Work out the finished part from the listing and answer in its coordinate system (mm). Round coordinates to 2 decimals unless told otherwise and drop trailing zeros. Write each loop counter-clockwise with the first axis right and the second up, starting at its lowest first coordinate (ties: lowest second). Pieces come first, ordered by that corner, then holes.
1. Find section B-B (x = 14). Write down the section's boundary in (y, z), and give its area (3 significant figures).
2. Straight lines are drawn through the part: probe 1 along Y at (x, z) = (0, -0.9); probe 2 along Y at (x, z) = (9, 0.9); probe 3 along Y at (x, z) = (-5.5, -1.25). For each, find the intervals that lie inside material, in ascending order.
3. Find section A-A (z = -0.25). Write down the section's boundary in (x, y).
4. Flat-ended cylindrical pins translate along their axes: pin 1 Ø1.5 at (y, z) = (-187.5, -0.5) entering from +X; pin 2 Ø1 at (x, z) = (7.5, 0.5) entering from +Y; pin 3 Ø1.5 at (x, z) = (12, 0) entering from -Y. Find the tip coordinate at first contact, or state that the pin passes through.
Autodesk Inventor part; units mm, degrees
ref_plane "YZ Plane" through (0, 0, 0) normal (1, 0, 0) x (0, 1, 0)
ref_plane "XZ Plane" through (0, 0, 0) normal (0, 1, 0) x (-1, 0, 0)
ref_plane "XY Plane" through (0, 0, 0) normal (0, 0, 1) x (1, 0, 0)
sketch "Sketch1" plane through (0, 0, 0) normal (0, 0, 1) x (1, 0, 0)
  line L0 (-25, 0) -> (25, 0)
  line L1 (25, 0) -> (25, -830)
  line L2 (25, -830) -> (-25, -830)
  line L3 (-25, -830) -> (-25, 0)
  line L4 (25, -830) -> (-25, -793.2713)
  line L5 (25, 0) -> (-25, -68.0668)
  point P0 (0, 0)
  point P1 (0, 0)
  point P2 (25, -1153.2713)
  dimension "d0" = 50
  dimension "d1" = 830
  dimension "d5" = 53.7
  dimension "d6" = 53.7
extrude "Plate1" add sketch "Sketch1" along normal mid plane 3 contours L1 L4 L3 L5
chamfer "Corner Chamfer1" distance 3 angle 45 1 edges at (25, -830, 0)
chamfer "Corner Chamfer2" distance 3 angle 45 1 edges at (25, 0, 0)
fillet "Corner Round1" radius 6 1 edges at (-25, -68.0668, 0)
fillet "Corner Round2" radius 6 1 edges at (-25, -793.2713, 0)
sketch "Sketch2" plane through (0, 0, 1.5) normal (0, 0, 1) x (1, 0, 0)
  line L0 (25, -186.5) -> (-1, -186.5)
  line L1 (-1, -186.5) -> (-1, -189.5)
  line L2 (-1, -189.5) -> (25, -189.5)
  line L3 (25, -189.5) -> (25, -186.5)
  line L4 (25, -3) -> (25, -827)
  point P0 (0, 0)
  point P1 (25, -188)
  dimension "d15" = 188
  dimension "d16" = 26
  dimension "d17" = 3
extrude "Extrusion1" cut sketch "Sketch2" against normal through all
pattern_linear "Rectangular Pattern1" count 2 spacing 377 along (0, -1, 0) of "Extrusion1"
equation "\"d6\" = d5"
equation "\"d2\" = Thickness"
equation "\"BendReliefWidth\" = Thickness"
equation "\"BendReliefDepth\" = 0.5 * Thickness"
equation "\"CornerReliefSize\" = 4 * Thickness"
equation "\"MinimumRemnant\" = 2 * Thickness"
equation "\"TransitionRadius\" = BendRadius"
equation "\"JacobiRadiusSize\" = BendRadius"
equation "\"GapSize\" = Thickness"
properties part number "MSC 0163 stringer cone exit back" material "Stainless Steel"
Worked answers:
1. outline: (-821.92, -1.5) - (-566.5, -1.5) - (-566.5, 1.5) - (-821.92, 1.5) - close; (-563.5, -1.5) - (-189.5, -1.5) - (-189.5, 1.5) - (-563.5, 1.5) - close; (-186.5, -1.5) - (-14.97, -1.5) - (-14.97, 1.5) - (-186.5, 1.5) - close
1. area: 2,400 mm2
2. probe 1: y = -811.64 to -566.5, -563.5 to -189.5, -186.5 to -34.03
2. probe 2: y = -818.25 to -566.5, -563.5 to -189.5, -186.5 to -21.78
2. probe 3: y = -807.6 to -41.52
3. outline: (-25, -790.23) arc R6 ccw to (-22.55, -795.07) - (22.58, -828.22) - (25, -827) - (25, -566.5) - (-1, -566.5) - (-1, -563.5) - (25, -563.5) - (25, -189.5) - (-1, -189.5) - (-1, -186.5) - (25, -186.5) - (25, -3) - (23.22, -2.42) - (-23.84, -66.48) arc R6 ccw to (-25, -70.03) - close
4. pin 1: stops at x = -1
4. pin 2: stops at y = -23.14
4. pin 3: stops at y = -821
